Work out the finished part from the listing and answer in its coordinate system (mm). A direction names the side the tool comes from. Round coordinates to 2 decimals unless told otherwise and drop trailing zeros. Loops run counter-clockwise (first coordinate to the right, second up) from the corner with the lowest first, then second, coordinate; pieces in that order, holes last. Notation, with made-up numbers: (46.25, 40) - (101.25, 40) arc R12 ccw to (101.25, 58) - close; hole circle Ø7 at (45, -4.75). An arc over 180 degrees is marked (long way). Use CSV: the item, a comma, the result in double quotes. Start each with the question number.
from build123d import *

# Parameters (mm, degrees)
F0_W     = 115
F0_H     = 15
F0_R     = 3.15
F1_DEPTH = 3
F2_W     = 25
F2_H     = 15
F4_DEPTH = 3
F3_W     = 25
F3_H     = 15
F5_DEPTH = 3
F6_R     = 5


with BuildPart() as f1:
    # F0 (on Front) → F1 (new body, symmetric)
    with BuildSketch(Plane.XZ):
        with Locations((-1.0412013265, -7.5)):
            Rectangle(F0_W, F0_H)
        with Locations((-51.0412013265, -7.5)):
            Circle(F0_R, mode=Mode.SUBTRACT)
        with Locations((48.9587986735, -7.5)):
            Circle(F0_R, mode=Mode.SUBTRACT)
    extrude(amount=F1_DEPTH, both=True)

    # F2 (on Front) → F4 (cut)
    with BuildSketch(Plane.XZ):
        with Locations((-46.0412013265, -7.5)):
            Rectangle(F2_W, F2_H)
    extrude(amount=-F4_DEPTH, mode=Mode.SUBTRACT)

    # F3 (on Front) → F5 (cut)
    with BuildSketch(Plane.XZ):
        with Locations((43.9587986735, -7.5)):
            Rectangle(F3_W, F3_H)
    extrude(amount=F5_DEPTH, mode=Mode.SUBTRACT)

    # F6
    f6_edges = [f1.edges().sort_by_distance(p)[0] for p in [
        (-58.541201, -1.5, 0),
        (-58.541201, -1.5, -15),
        (56.458799, 1.5, -15),
        (56.458799, 1.5, 0),
    ]]
    fillet(f6_edges, radius=F6_R)


solid = f1.part
Item 1: Find the intervals of material crossed by probe 1 along X at (y, z) = (1.1, -7.5); probe 2 along X at (y, z) = (-0.75, -7.5); probe 3 along Y at (x, z) = (46, -11.5), in increasing order. Write a range as [from, to].
Item 2: A cutting plane is placed at C-C (z = -2.5). Determine the outline of the cut face in (x, y), plus the area to 3 significant figures.
Item 3: Each of these flat-tipped pins is pushed along its axis until it touches: pin 1 Ø2 at (y, z) = (1.5, -13) entering from +X; pin 2 Ø2 at (y, z) = (-0.5, -11.5) entering from +X; pin 3 Ø4.5 at (x, z) = (-41.5, -9.5) entering from +Y. Where does it stop, or does it pass through?
Item 4: A cutting plane is placed at A-A (z = -7.5). Determine the outline of the cut face in (x, y), plus the area to 3 significant figures.
Item 5: A cutting plane is placed at B-B (y = 1.15). Determine the outline of the cut face in (x, z), plus the area to 3 significant figures.
Item 6: A cutting plane is placed at D-D (x = -38). Determine the outline of the cut face in (y, z), plus the area to 3 significant figures.
Item 7: Which of the six approach directions +Z, -Z, +X, -X, +Y, -Y give full straight-line access (tool end or side, diameter ignored) to faces 4 (the flat face through (-46, 0, -7)), 5 (the flat face through (44, 0, -7)), 6 (the flat face through (-58.541, -2, -8))?
Item 8: The mould has two halves that part along X. Classify faces 1 (the cylindrical face through (46.64, 1.52, -5.37)), 2 (the flat face through (11, 3, -7)), 3 (the cylindrical face through (-57.115, -1.479, -1.504)): pulls with the +X half, pulls with the -X half, needs draft (parallel to the pull), parting line crosses it, or undercut.
Result sheet:
1,probe 1,"[-33.54, 45.81], [52.11, 56.46]"
1,probe 2,"[-58.54, -54.19], [-47.89, 31.46]"
1,probe 3,"[0, 3]"
2,outline,"(-57.87, -3) - (31.46, -3) - (31.46, 0) - (55.79, 0) - (55.79, 3) - (-33.54, 3) - (-33.54, 0) - (-57.87, 0) - close"
2,area,"536 mm^2"
3,pin 1,"x = 56.04"
3,pin 2,"x = 56.42"
3,pin 3,"y = 0"
4,outline,"(-58.54, -3) - (-54.19, -3) - (-54.19, 0) - (-58.54, 0) - close; (-47.89, -3) - (31.46, -3) - (31.46, 0) - (45.81, 0) - (45.81, 3) - (-33.54, 3) - (-33.54, 0) - (-47.89, 0) - close; (52.11, 0) - (56.46, 0) - (56.46, 3) - (52.11, 3) - close"
4,area,"502 mm^2"
5,outline,"(-33.54, -15) - (51.46, -15) arc R5 ccw to (56.46, -10) - (56.46, -5) arc R5 ccw to (51.46, 0) - (-33.54, 0) - close; hole circle Ø6.3 at (48.96, -7.5)"
5,area,"1,310 mm^2"
6,outline,"(-3, -15) - (0, -15) - (0, 0) - (-3, 0) - close"
6,area,"45.0 mm^2"
7,face 4,"+Z, -Z, -X, +Y"
7,face 5,"+Z, -Z, +X, -Y"
7,face 6,"+Z, -Z, -X, +Y, -Y"
8,face 1,"undercut"
8,face 2,"needs draft"
8,face 3,"pulls with the -X half"
